from build123d import *

# Parameters (mm, degrees)
SKETCH_1_R          = 15
EXTRUDE_1_DEPTH     = 34
SKETCH_2_R          = 12
EXTRUDE_2_DEPTH     = 8
SKETCH_3_R          = 9
EXTRUDE_3_DEPTH     = 3
SKETCH_4_R          = 10
EXTRUDE_4_DEPTH     = 15
SKETCH_5_R          = 9
EXTRUDE_5_DEPTH     = 16
EXTRUDE_START       = 8
SKETCH_6_R          = 12
EXTRUDE_6_DEPTH     = 8
EXTRUDE_START_2     = 3
SKETCH_7_R          = 9
EXTRUDE_7_DEPTH     = 3
EXTRUDE_START_3     = 15
SKETCH_8_R          = 10
EXTRUDE_8_DEPTH     = 15
SKETCH_9_R          = 7
EXTRUDE_9_DEPTH     = 10
SKETCH_10_R         = 5.5
EXTRUDE_10_DEPTH    = 3.5
CUT_EXTRUDE_START   = 7.7
CUT_EXTRUDE_1_DEPTH = 3.5


# Read off the part's stored shape, not the designer's step: the loft step
with BuildPart() as part:
    # Sketch 1 → Extrude 1 (new body)
    with BuildSketch(Plane(origin=(0, 0, 0), x_dir=(0, 0, -1), z_dir=(1, 0, 0))):
        Circle(SKETCH_1_R)
    extrude(amount=EXTRUDE_1_DEPTH)

    # Sketch 2 → Extrude 2 (add)
    with BuildSketch(Plane(origin=(34, 0, 0), x_dir=(0, 0, -1), z_dir=(1, 0, 0))):
        Circle(SKETCH_2_R)
    extrude(amount=EXTRUDE_2_DEPTH)

    # Sketch 3 → Extrude 3 (add)
    with BuildSketch(Plane(origin=(42, 0, 0), x_dir=(0, 0, -1), z_dir=(1, 0, 0))):
        Circle(SKETCH_3_R)
    extrude(amount=EXTRUDE_3_DEPTH)

    # Sketch 4 → Extrude 4 (add)
    with BuildSketch(Plane(origin=(45, 0, 0), x_dir=(0, 0, -1), z_dir=(1, 0, 0))):
        Circle(SKETCH_4_R)
    extrude(amount=EXTRUDE_4_DEPTH)

    # Sketch 5 → Extrude 5 (add)
    with BuildSketch(Plane(origin=(60, 0, 0), x_dir=(0, 0, -1), z_dir=(1, 0, 0))):
        Circle(SKETCH_5_R)
    extrude(amount=EXTRUDE_5_DEPTH)

    # Sketch 6 → Extrude 6 (add)
    with BuildSketch(Plane.ZY.offset(EXTRUDE_START)):
        with Locations(Location((0, 0, 0), (0, 0, 180))):
            Circle(SKETCH_6_R)
    extrude(amount=-EXTRUDE_6_DEPTH)

    # Sketch 7 → Extrude 7 (add)
    with BuildSketch(Plane.ZY.offset(8).offset(EXTRUDE_START_2)):
        with Locations(Location((0, 0, 0), (0, 0, 180))):
            Circle(SKETCH_7_R)
    extrude(amount=-EXTRUDE_7_DEPTH)

    # Sketch 8 → Extrude 8 (add)
    with BuildSketch(Plane.ZY.offset(11).offset(EXTRUDE_START_3)):
        with Locations(Location((0, 0, 0), (0, 0, 180))):
            Circle(SKETCH_8_R)
    extrude(amount=-EXTRUDE_8_DEPTH)



with BuildPart() as body_2:
    # Sketch 9 → Extrude 9 (new body)
    with BuildSketch(Plane(origin=(130, 0, 0), x_dir=(0, 0, -1), z_dir=(1, 0, 0))):
        Circle(SKETCH_9_R)
    extrude(amount=EXTRUDE_9_DEPTH)

    # Sketch 10 → Extrude 10 (add)
    with BuildSketch(Plane.ZY.offset(-130)):
        with Locations(Location((0, 0, 0), (0, 0, 180))):
            Circle(SKETCH_10_R)
    extrude(amount=EXTRUDE_10_DEPTH)


with BuildPart() as part_1:
    add(part.part)

    add(body_2.part)  # Loft 1 merges body 2
    # Loft 1 outline → Loft 1 (revolve)
    with BuildSketch(Plane.YX):
        Polygon((8, 126.5), (0, 126.5), (0, 76), (9, 76), align=None)
    revolve(axis=Axis((0, 0, 0), (1, 0, 0)))

    # Sketch 12 → Cut-Extrude 1 (cut)
    with BuildSketch(Plane(origin=(0, 0, 0), x_dir=(1, 0, 0), z_dir=(0, 1, 0)).offset(CUT_EXTRUDE_START)):
        with BuildLine():
            Line((82, -3), (106, -3))
            ThreePointArc((106, -3), (109, 0), (106, 3))
            Line((106, 3), (82, 3))
            ThreePointArc((82, 3), (79, 0), (82, -3))
        make_face()
    extrude(amount=CUT_EXTRUDE_1_DEPTH, mode=Mode.SUBTRACT)


solid = part_1.part
Here's how the part is built. I have some questions about the finished solid (model axes, mm). A direction names the side the tool comes from. Give positions to 0.01 mm unless a question says otherwise; leave off trailing zeros. Order: outer loops, then holes, each group sorted by start corner. A loop starts at its lowest first (then second) coordinate and runs counter-clockwise, first axis right, second up. Notation, with made-up numbers: M 53,-35.5 L 66,-35.5 A18 ccw 66,-21.5 Z; hole C 33.5,41.25 d8. An arc over 180 degrees is marked long. Answer as a JSON object with one key per item and string values. Group by question number.
1) Please list where these lines run through material, in increasing order: L1, parallel to X at y = 7.5, z = 5.25; L2, parallel to Y at x = 33, z = -12. Write a range as [from, to].
2) I'm going to push flat-ended pins straight in: pin 1 Ø8 at (x, y) = (93, 6) entering from +Z; pin 2 Ø2 at (x, y) = (111.5, 1) entering from -Z; pin 3 Ø8 at (x, z) = (40.5, -7) entering from +Y. Where does each tip first touch, or does it pass through?
3) Suppose I cut it at C-C, the plane x = 96. Write out the boundary of the cut face in (y, z), plus the area to 3 significant figures.
4) Suppose I cut it at A-A, the plane x = 47. Write out the boundary of the cut face in (y, z).
5) We'd pull the mould along X, two halves only. Please class faces 1 (the flat face through (42, 9, -2)), 2 (the cylindrical face through (134.93, -2.681, -6.466)), 3 (the flat face through (60, 2, 9)): pulls with the +X half, pulls with the -X half, needs draft (parallel to the pull), parting line crosses it, or undercut.
6) On a 3-axis mill with a long thin cutter (end or side, diameter ignored), from which of +Z, -Z, +X, -X, +Y, -Y can I reach the whole of each face in a straight line? I mean faces 4 (the cylindrical face through (37.94, 0.53, 11.99)), 5 (the cylindrical face through (43.479, 8.923, 1.172)), 6 (the cylindrical face through (-4.056, -3.604, -11.446)). Say none if no direction works.
7) Suppose I cut it at B-B, the plane x = 25. Write out the boundary of the cut face in (y, z), plus the area to 3 significant figures.
Results found:
{
 "1": {"L1": "[-26, -11], [-8, 42], [45, 60]", "L2": "[-9, 9]"},
 "2": {"pin 1": "z = 8.43", "pin 2": "z = -8.31", "pin 3": "y = 11.62"},
 "3": {"outline": "M 7.7,-3 L 7.7,3 L 8.06,3 A8.6 ccw long 8.06,-3 Z", "area": "228 mm²"},
 "4": {"outline": "C 0,0 d20"},
 "5": {"face 1": "undercut", "face 2": "needs draft", "face 3": "pulls with the +X half"},
 "6": {"face 4": "+X", "face 5": "none", "face 6": "-X"},
 "7": {"outline": "C 0,0 d30", "area": "707 mm²"}
}
